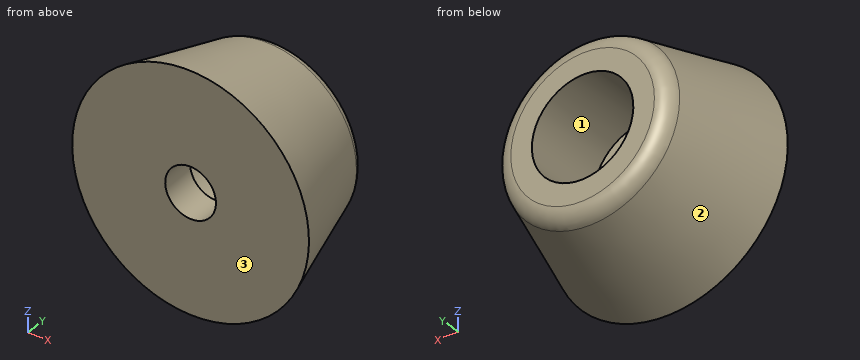
from build123d import *


with BuildPart() as part:
    # Croquis1 → Revolución1 (revolve)
    with BuildSketch(Plane.XY, mode=Mode.PRIVATE) as revoluci_n1_sk:
        with BuildLine():
            Line((-7, 0), (-1.5, 0))
            Line((-1.5, 0), (-1.5, 2))
            Line((-1.5, 2), (-3, 2))
            Line((-3, 2), (-3, 7))
            Line((-3, 7), (-4.245698587, 7))
            ThreePointArc((-4.245698587, 7), (-4.8478941, 6.798348648), (-5.207222535, 6.274721128))
            Line((-5.207222535, 6.274721128), (-7, 0))
        make_face()
    revolve(revoluci_n1_sk.sketch.rotate(Axis((0, 0, 0), (0, 1, 0)), 270), axis=Axis((0, 0, 0), (0, 1, 0)))


solid = part.part
Model file for the job. Use its own axes, mm. Face numbers are marked on the shaded views. Give positions to 0.01 mm unless a question says otherwise; leave off trailing zeros. Order: outer loops, then holes, each group sorted by start corner. A loop starts at its lowest first (then second) coordinate and runs counter-clockwise, first axis right, second up. Notation, with made-up numbers: (20.25, -14.75) - (34.25, -14.75) arc R5 cw to (34.25, -9.75) - close; hole circle Ø5 at (68, 40.5). An arc over 180 degrees is marked (long way). One line per item, written item: value.
Item 1: Wall check: line 1 (X direction, y = 4, z = 0.75); line 2 (Z direction, x = -2.75, y = 3.5); line 3 (X direction, y = 5.6, z = 0). Give the ranges that are in metal, low to high.
Response values:
line 1: -5.81 to -2.9, 2.9 to 5.81
line 2: -5.33 to -1.2, 1.2 to 5.33
line 3: -5.4 to -3, 3 to 5.4
Item 2: Slice it at B-B (y = 1.75). List the corners of the cut face in (x, z), then the cut area to 3 significant figures.
Response values:
outline: circle Ø13 at (0, 0); hole circle Ø3 at (0, 0)
area: 126 mm2
Item 3: Pin check, flat tips, straight feed: pin 1 Ø4 at (x, y) = (-1, 5.5) entering from -Z; pin 2 Ø1 at (x, y) = (-3.5, 5.5) entering from -Z; pin 3 Ø2 at (x, z) = (-4, -4) entering from +Y. Stop position of each tip, or through.
Response values:
pin 1: z = -5.96
pin 2: z = -4.57
pin 3: y = 6.91
Item 4: Slice it at C-C (y = 5). List the corners of the cut face in (x, z).
Response values:
outline: circle Ø11.14 at (0, 0); hole circle Ø6 at (0, 0)
Item 5: Slice it at A-A (z = 0). List the corners of the cut face in (x, y), then the cut area to 3 significant figures.
Response values:
outline: (-7, 0) - (-1.5, 0) - (-1.5, 2) - (-3, 2) - (-3, 7) - (-4.25, 7) arc R1 ccw to (-5.21, 6.27) - close; (1.5, 0) - (7, 0) - (5.21, 6.27) arc R1 ccw to (4.25, 7) - (3, 7) - (3, 2) - (1.5, 2) - close
area: 47.8 mm2
Item 6: Two-plate mould, pull along Z, no slides. Class the marked faces 1, 2 and 3: released by +Z, released by -Z, zero draft, split by the parting line, or undercut.
Response values:
face 1: undercut
face 2: split by the parting line
face 3: zero draft
